Design review of the part built by this model. Coordinates are the model's own, in mm. Round coordinates to 2 decimals unless told otherwise and drop trailing zeros. Order: outer loops, then holes, each group sorted by start corner. A loop starts at its lowest first (then second) coordinate and runs counter-clockwise, first axis right, second up. Notation, with made-up numbers: (40, 3.25) - (89, 3.25) arc R14 ccw to (89, 21.25) - close; hole circle Ø7 at (16.5, 29.5). An arc over 180 degrees is marked (long way). Use CSV: the item, a comma, the result in double quotes.
from build123d import *

# Parameters (mm, degrees)
SKETCH1_R           = 3.375
BOSS_EXTRUDE2_DEPTH = 38.1
BOSS_EXTRUDE3_REACH = 82.814
SKETCH6_W           = 38.1
SKETCH6_H           = 36.425
SKETCH10_R          = 2
CUT_EXTRUDE6_DEPTH  = 8
CHAMFER1_SIZE       = 1
CUT_EXTRUDE11_DEPTH = 6.35
SKETCH16_R          = 2
CUT_EXTRUDE10_DEPTH = 5
SKETCH17_R          = 1
CUT_EXTRUDE12_DEPTH = 77.103956903
FILLET1_R           = 2


with BuildPart() as part:
    # Sketch1 → Boss-Extrude2 (new body)
    with BuildSketch(Plane(origin=(0, 0, 0), x_dir=(0, 0, -1), z_dir=(1, 0, 0))):
        with BuildLine():
            Line((61.825, 22.75), (0, 22.75))
            Line((0, 22.75), (0, 0))
            Line((0, 0), (0.0025, 0))
            ThreePointArc((0.0025, 0), (12.7025, -12.7), (25.4025, 0))
            Line((25.4025, 0), (36.4275, 0))
            ThreePointArc((36.4275, 0), (49.253496032, -12.699374985), (61.825, 0.251979662))
            Line((61.825, 0.251979662), (61.825, 22.75))
        make_face()
        with Locations(Location((49.1275, 0, 0), (0, 0, 180))):
            Circle(SKETCH1_R, mode=Mode.SUBTRACT)
        with Locations(Location((12.7025, 0, 0), (0, 0, 180))):
            Circle(SKETCH1_R, mode=Mode.SUBTRACT)
    extrude(amount=BOSS_EXTRUDE2_DEPTH)

    # Sketch6 → Boss-Extrude3 (add, up to next)
    with BuildSketch(Plane(origin=(0, -12.7, 0), x_dir=(-1, 0, 0), z_dir=(0, -1, 0)), mode=Mode.PRIVATE) as boss_extrude3_sk1:
        with Locations((-19.05, 30.915)):
            Rectangle(SKETCH6_W, SKETCH6_H)
    boss_extrude3_tool1 = extrude(boss_extrude3_sk1.sketch, amount=-BOSS_EXTRUDE3_REACH, mode=Mode.PRIVATE) - part.part
    add(boss_extrude3_tool1.solids().sort_by_distance((19.05, -12.7, -30.915))[0])

    # Sketch10 → Cut-Extrude6 (cut)
    with BuildSketch(Plane.XY):
        with Locations((9.525, 14.153125)):
            Circle(SKETCH10_R)
        with Locations((28.575, 14.153125)):
            Circle(SKETCH10_R)
    extrude(amount=-CUT_EXTRUDE6_DEPTH, mode=Mode.SUBTRACT)

    # Chamfer1
    chamfer1_edges = [part.edges().sort_by_distance(p)[0] for p in [
        (0, 0, -16.0775),
        (0, 0, -52.5025),
        (38.1, 0, -16.0775),
        (38.1, 0, -52.5025),
    ]]
    chamfer(chamfer1_edges, length=CHAMFER1_SIZE)

    # Sketch15 → Cut-Extrude11 (cut)
    with BuildSketch(Plane(origin=(0, 22.75, 0), x_dir=(1, 0, 0), z_dir=(0, 1, 0))):
        Polygon((12.5, 31.95), (0, 31.95), (0, 29.88), (15.26, 29.88), (15.26, 61.825), (12.5, 61.825), align=None)
        Polygon((25.6, 61.825), (22.84, 61.825), (22.84, 29.88), (38.1, 29.88), (38.1, 31.95), (25.6, 31.95), align=None)
    extrude(amount=-CUT_EXTRUDE11_DEPTH, mode=Mode.SUBTRACT)

    # Sketch16 → Cut-Extrude10 (cut)
    with BuildSketch(Plane(origin=(0, 22.75, 0), x_dir=(1, 0, 0), z_dir=(0, 1, 0))):
        with Locations(Location((32.1, 41.225, 0), (0, 0, 270))):
            Circle(SKETCH16_R)
        with BuildLine():
            ThreePointArc((21.05, 26.985), (20.464213562, 28.399213562), (19.05, 28.985))
            Line((19.05, 28.985), (19.05, 24.985))
            ThreePointArc((19.05, 24.985), (20.464213562, 25.570786438), (21.05, 26.985))
        make_face()
        with BuildLine():
            Line((19.05, 24.985), (19.05, 28.985))
            ThreePointArc((19.05, 28.985), (17.05, 26.985), (19.05, 24.985))
        make_face()
        with Locations(Location((6, 41.225, 0), (0, 0, 270))):
            Circle(SKETCH16_R)
        with Locations(Location((10, 20, 0), (0, 0, 270))):
            Circle(SKETCH16_R)
        with Locations(Location((20, 10, 0), (0, 0, 270))):
            Circle(SKETCH16_R)
    extrude(amount=-CUT_EXTRUDE10_DEPTH, mode=Mode.SUBTRACT)

    # Sketch17 → Cut-Extrude12 (cut, through all)
    with BuildSketch(Plane(origin=(38.1, 0, 0), x_dir=(0, 0, -1), z_dir=(1, 0, 0))):
        with Locations((12.7025, -3.375)):
            Circle(SKETCH17_R)
        with Locations((49.1275, -3.375)):
            Circle(SKETCH17_R)
    extrude(amount=-CUT_EXTRUDE12_DEPTH, mode=Mode.SUBTRACT)

    # Fillet1
    fillet1_edges = [part.edges().sort_by_distance(p)[0] for p in [
        (15.26, 19.575, -29.88),
        (12.5, 19.575, -31.95),
        (22.84, 19.575, -29.88),
        (25.6, 19.575, -31.95),
    ]]
    fillet(fillet1_edges, radius=FILLET1_R)


solid = part.part
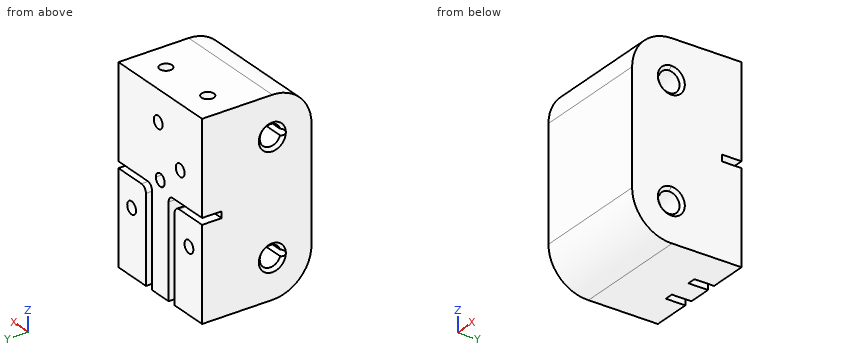
1) We need section C-C (y = -10). Give the boundary of the cut face in (x, z), then the cut area to 3 significant figures.
Data:
outline,"(0, -56.96) - (38.1, -56.96) - (38.1, -4.87) - (0, -4.87) - close"
area,"1,980 mm2"
2) We need section B-B (z = -55.5). Give the boundary of the cut face in (x, y), then the cut area to 3 significant figures.
Data:
outline,"(0, -10.99) - (38.1, -10.99) - (38.1, 22.75) - (25.6, 22.75) - (25.6, 16.4) - (22.84, 16.4) - (22.84, 22.75) - (15.26, 22.75) - (15.26, 16.4) - (12.5, 16.4) - (12.5, 22.75) - (0, 22.75) - close"
area,"1,250 mm2"
3) We need section A-A (x = 6). Give the number of separate pieces and of enclosed holes in the cut face, then the cut area to 3 significant figures.
Data:
separate pieces,"1"
enclosed holes,"2"
area,"2,010 mm2"
4) Insertion check: pin 1 Ø3 at (x, y) = (28.58, 14.15) entering from +Z; pin 2 Ø7 at (x, y) = (5.5, 19.5) entering from -Z (3 decimals); pin 3 Ø2 at (x, z) = (18, -10) entering from -Y. Each pin has a flat end and moves straight along its axis. Give the tip position at first contact, or say it passes through.
Data:
pin 1,"stops at z = -8"
pin 2,"stops at z = -61.825"
pin 3,"stops at y = -12.59"
5) To check wall thickness, follow L1, parallel to Z at x = 36.5, y = 9 (3 decimals); L2, parallel to Z at x = 8, y = 13.5 (3 decimals); L3, parallel to Y at x = 23, z = -51. State the ranges of each line that lie inside material, in increasing order. Write a range as from..to.
Data:
L1,"z = -61.825..0"
L2,"z = -61.825..-8"
L3,"y = -12.56..-2.81, 2.81..16.4"
